Part model, mm, in its own coordinate system. A direction names the side the tool comes from. Give positions to 0.01 mm unless a question says otherwise; leave off trailing zeros. Loops run counter-clockwise (first coordinate to the right, second up) from the corner with the lowest first, then second, coordinate; pieces in that order, holes last. Notation, with made-up numbers: M -39,56.5 L 14,56.5 A15 ccw 14,68.5 Z; hole C 59,81.25 d6. An arc over 180 degrees is marked long. Answer in a Markdown table with one row per item.
Autodesk Inventor part; units mm, degrees
ref_plane "YZ Plane" through (0, 0, 0) normal (1, 0, 0) x (0, 1, 0)
ref_plane "XZ Plane" through (0, 0, 0) normal (0, 1, 0) x (-1, 0, 0)
ref_plane "XY Plane" through (0, 0, 0) normal (0, 0, 1) x (1, 0, 0)
sketch "Эскиз1" plane through (0, 0, 0) normal (0, 1, 0) x (-1, 0, 0)
  line L0 (0, 0) -> (58, 0)
  line L1 (58, 0) -> (58, 65)
  line L2 (58, 65) -> (38, 86.8785)
  line L3 (0, 0) -> (0, 102)
  line L4 (0, 102) -> (38, 102)
  line L5 (38, 102) -> (38, 86.8785)
  line L6 (0, 0) -> (49, 0)
  line L7 (49, 0) -> (49, 10)
  line L8 (49, 10) -> (49, 60)
  dimension "d8" = 58
  dimension "d9" = 65
  dimension "d10" = 102
  dimension "d11" = 38
  dimension "d12" = 49
  dimension "d13" = 10
  dimension "d14" = 50
extrude "Выдавливание1" add sketch "Эскиз1" along normal blind 12
sketch "Эскиз3" plane through (0, 12, 0) normal (0, 1, 0) x (1, 0, 0)
  line L0 (-38, -102) -> (0, -102)
  line L1 (-38, -102) -> (-38, -89)
  line L2 (-38, -86.8785) -> (-38, -102)
  line L3 (-38, -89) -> (0, -89)
  line L4 (0, -89) -> (0, -102)
  point P0 (0, 0)
  dimension "d17" = 13
extrude "Выдавливание2" add sketch "Эскиз3" against normal blind 38
sketch "Эскиз4" plane through (0, 12, 0) normal (0, 1, 0) x (1, 0, 0)
  line L0 (0, 0) -> (-58, 0)
  line L1 (0, 0) -> (-49, 0)
  line L2 (-49, 0) -> (-49, -10)
  line L3 (-49, -10) -> (-49, -60)
  dimension "d20" = 49
  dimension "d21" = 10
  dimension "d22" = 50
hole "Отверстие1" at (-49, 12, 60) at (-49, 12, 10) direction (0, -1, 0) diameter 9 end through all counterbore diameter 14 counterbore depth 9
sketch "Эскиз6" plane through (-38, 12, 102) normal (0, 0, 1) x (1, 0, 0)
  line L0 (38, -37.7549) -> (10.0011, -38)
  line L1 (0, -38) -> (38, -38)
  line L2 (10.0011, -38) -> (10.0011, -27)
  point P0 (38, -12)
  dimension "d39" = 28
  dimension "d40" = 11
hole "Отверстие3" at (-27.9989, -15, 102) direction (0, 0, -1) diameter 10 end through all
mirror "Зеркальное отражение1" about plane through (0, 0, 102) normal (1, 0, 0) of "Выдавливание2", "Выдавливание1", "Отверстие1", "Отверстие3"
thread "Резьба1"
thread "Резьба2"
chamfer "Фаска1" distance 1.6 angle 45 2 edges at (27.9989, -10, 102) (-27.9989, -10, 102)
chamfer "Фаска2" distance 3 angle 45 1 edges at (0, 12, 102)
chamfer "Фаска3" distance 2 angle 45 2 edges at (58, 6, 0) (-58, 6, 0)
properties part number "Крышка-6"
(1) Saw through at B-B (z = 60). Write the cut outline in (x, y).
Recorded:
| item | result |
|---|---|
| outline | M -58,0 L -53.5,0 L -53.5,3 L -56,3 L -56,12 L -58,12 Z; M -44.5,0 L 44.5,0 L 44.5,3 L 42,3 L 42,12 L -42,12 L -42,3 L -44.5,3 Z; M 53.5,0 L 58,0 L 58,12 L 56,12 L 56,3 L 53.5,3 Z |
(2) Saw through at C-C (x = -18). Write the cut outline in (y, z).
Recorded:
| item | result |
|---|---|
| outline | M -26,89 L 0,89 L 0,0 L 12,0 L 12,99 L 9,102 L -26,102 Z |
(3) Saw through at A-A (y = -15). Write the cut outline in (x, z), plus the area to 3 significant figures.
Recorded:
| item | result |
|---|---|
| outline | M -38,89 L -33,89 L -33,100.4 L -34.6,102 L -38,102 Z; M -23,89 L 23,89 L 23,100.4 L 21.4,102 L -21.4,102 L -23,100.4 Z; M 33,89 L 38,89 L 38,102 L 34.6,102 L 33,100.4 Z |
| area | 723 mm^2 |
(4) Which spindle directions (+Z, -Z, +X, -X, +Y, -Y) get a long thin tool onto all of the face, cutting with end or side? Do faces 4 (the face through (1, 0, 45)), 5 (the face through (-1, 11, 100)), 6 (the face through (49, 3, 5)). Say none if no direction does.
Recorded:
| item | result |
|---|---|
| face 4 | -Z, +X, -X, -Y |
| face 5 | +Z, +X, -X, +Y |
| face 6 | +Y |
(5) Drill centre lines: line 1 along X through (y, z) = (-15, 93); line 2 along X through (y, z) = (2.05, 10); line 3 along Z through (x, y) = (-49, 0.7). Where is each one in solid material? Low to high.
Recorded:
| item | result |
|---|---|
| line 1 | x = -38 to -33, -23 to 23, 33 to 38 |
| line 2 | x = -58 to -53.5, -44.5 to 44.5, 53.5 to 58 |
| line 3 | z = 0 to 5.5, 14.5 to 55.5, 64.5 to 74.85 |
(6) Saw through at D-D (x = -49). Write the cut outline in (y, z), plus the area to 3 significant figures.
Recorded:
| item | result |
|---|---|
| outline | M 0,0 L 12,0 L 12,3 L 3,3 L 3,5.5 L 0,5.5 Z; M 0,14.5 L 3,14.5 L 3,17 L 12,17 L 12,53 L 3,53 L 3,55.5 L 0,55.5 Z; M 0,64.5 L 3,64.5 L 3,67 L 12,67 L 12,74.85 L 0,74.85 Z |
| area | 592 mm^2 |
(7) Pull direction X, two halves, no side cores. Call faces 1 (the face through (-38, -7, 95)), 2 (the face through (-44, 3, 60)), 3 (the face through (47.86, 5.92, 76.09)): +X half, -X half, draft (parallel to the pull), parting line (faces both ways), or undercut.
Recorded:
| item | result |
|---|---|
| face 1 | -X half |
| face 2 | undercut |
| face 3 | +X half |
(8) Pin check, flat tips, straight feed: pin 1 Ø11.5 at (x, z) = (-49, 10) entering from -Y; pin 2 Ø12 at (y, z) = (-1, 92) entering from -X; pin 3 Ø12 at (y, z) = (-8.5, 91) entering from +X; pin 4 Ø11 at (x, z) = (51.5, 61) entering from +Y. Stop position of each tip, or through.
Recorded:
| item | result |
|---|---|
| pin 1 | stops at y = 0 |
| pin 2 | stops at x = -38.73 |
| pin 3 | stops at x = 38 |
| pin 4 | stops at y = 12 |
